Here's how the part is built. I have some questions about the finished solid (model axes, mm). Face numbers are marked on the shaded views. A direction names the side the tool comes from. Round coordinates to 2 decimals unless told otherwise and drop trailing zeros. Loops run counter-clockwise (first coordinate to the right, second up) from the corner with the lowest first, then second, coordinate; pieces in that order, holes last. Notation, with made-up numbers: (-11, 20) -> (19, 20) arc R26 ccw to (19, 57) -> close; hole circle Ø1 at (59.25, 8). An arc over 180 degrees is marked (long way). Use one line per item in the form item = value. Start each with the question number.
Item 1: If we section it at D-D (z = 210.5): Write out the boundary of the cut face in (x, y) (1 decimal).
Item 2: I'm going to push flat-ended pins straight in: pin 1 Ø1.5 at (x, y) = (-221, -40.5) entering from +Z (3 decimals); pin 2 Ø2.5 at (x, y) = (186.5, -3.5) entering from +Z (3 decimals); pin 3 Ø3 at (x, y) = (74.5, 52.5) entering from -Z. Where does each tip first touch, or does it pass through?
Item 3: Thinking about a two-plate mould opening in Y: for the marked faces 3, 4, 5 and 6, which applies, released by +Y, released by -Y, zero draft, split by the parting line, or undercut?
Item 4: If we section it at C-C (x = -102): Write out the boundary of the cut face in (y, z) (1 decimal).
Item 5: If we section it at A-A (z = 130.5): State how many separate pieces and enclosed holes the cut face has, then the cut area to 3 significant figures.
Item 6: If we section it at B-B (y = 84): Write out the boundary of the cut face in (x, z) (3 decimals), then the cut area to 3 significant figures.
Item 7: If I drill on L1, parallel to X at y = 47, z = 183 (3 decimals); L2, parallel to Y at x = -155, z = 75.5; L3, parallel to Z at x = 12, y = 120 (3 decimals), over which ranges is the centre line in solid material (lowest first)? Write a range as [from, to].
Item 8: For the marked faces 1 and 2, which set-ups out of +Z, -Z, +X, -X, +Y, -Y let a thin tool reach every point of the face, with its end or its side?
```python
from build123d import *

# Parameters (mm, degrees)
SKETCH1_W           = 558.8
SKETCH1_H           = 315.575
SKETCH1_W_2         = 552.45
SKETCH1_H_2         = 309.225
SKETCH1_W_3         = 3.175
SKETCH1_W_4         = 89.789
SKETCH1_W_5         = 88.775
SKETCH1_W_6         = 88.644
BOSS_EXTRUDE1_DEPTH = 3.175
SKETCH2_W           = 558.8
SKETCH2_H           = 315.575
SKETCH2_W_2         = 552.45
SKETCH2_H_2         = 309.225
SKETCH2_W_3         = 3.175
BOSS_EXTRUDE2_DEPTH = 200.6
SKETCH3_W           = 558.8
SKETCH3_H           = 315.575
BOSS_EXTRUDE3_DEPTH = 32
CUT_EXTRUDE1_DEPTH  = 483.951127186


with BuildPart() as part:
    # Sketch1 → Boss-Extrude1 (new body)
    # profile 1 of 12: a face of its own
    with BuildSketch(Plane.XY):
        Rectangle(SKETCH1_W, SKETCH1_H)
        Rectangle(SKETCH1_W_2, SKETCH1_H_2, mode=Mode.SUBTRACT)
    # profile 2 of 12: a face of its own
    with BuildSketch(Plane.XY):
        with Locations((-185.8625, 0)):
            Rectangle(SKETCH1_W_3, SKETCH1_H_2)
    # profile 3 of 12: a face of its own
    with BuildSketch(Plane.XY):
        with Locations((-139.3805, 0)):
            Rectangle(SKETCH1_W_4, SKETCH1_H_2)
    # profile 4 of 12: a face of its own
    with BuildSketch(Plane.XY):
        with Locations((-231.8375, 0)):
            Rectangle(SKETCH1_W_5, SKETCH1_H_2)
    # profile 5 of 12: a face of its own
    with BuildSketch(Plane.XY):
        with Locations((-46.4165, 0)):
            Rectangle(SKETCH1_W_4, SKETCH1_H_2)
    # profile 6 of 12: a face of its own
    with BuildSketch(Plane.XY):
        with Locations((-92.8985, 0)):
            Rectangle(SKETCH1_W_3, SKETCH1_H_2)
    # profile 7 of 12: a face of its own
    with BuildSketch(Plane.XY):
        with Locations((46.5475, 0)):
            Rectangle(SKETCH1_W_4, SKETCH1_H_2)
    # profile 8 of 12: a face of its own
    with BuildSketch(Plane.XY):
        with Locations((0.0655, 0)):
            Rectangle(SKETCH1_W_3, SKETCH1_H_2)
    # profile 9 of 12: a face of its own
    with BuildSketch(Plane.XY):
        with Locations((139.5115, 0)):
            Rectangle(SKETCH1_W_4, SKETCH1_H_2)
    # profile 10 of 12: a face of its own
    with BuildSketch(Plane.XY):
        with Locations((93.0295, 0)):
            Rectangle(SKETCH1_W_3, SKETCH1_H_2)
    # profile 11 of 12: a face of its own
    with BuildSketch(Plane.XY):
        with Locations((231.903, 0)):
            Rectangle(SKETCH1_W_6, SKETCH1_H_2)
    # profile 12 of 12: a face of its own
    with BuildSketch(Plane.XY):
        with Locations((185.9935, 0)):
            Rectangle(SKETCH1_W_3, SKETCH1_H_2)
    extrude(amount=BOSS_EXTRUDE1_DEPTH)

    # Sketch2 → Boss-Extrude2 (add)
    # profile 1 of 6: a face of its own
    with BuildSketch(Plane.XY.offset(3.175)):
        Rectangle(SKETCH2_W, SKETCH2_H)
        Rectangle(SKETCH2_W_2, SKETCH2_H_2, mode=Mode.SUBTRACT)
    # profile 2 of 6: a face of its own
    with BuildSketch(Plane.XY.offset(3.175)):
        with Locations((-185.8625, 0)):
            Rectangle(SKETCH2_W_3, SKETCH2_H_2)
    # profile 3 of 6: a face of its own
    with BuildSketch(Plane.XY.offset(3.175)):
        with Locations((-92.8985, 0)):
            Rectangle(SKETCH2_W_3, SKETCH2_H_2)
    # profile 4 of 6: a face of its own
    with BuildSketch(Plane.XY.offset(3.175)):
        with Locations((0.0655, 0)):
            Rectangle(SKETCH2_W_3, SKETCH2_H_2)
    # profile 5 of 6: a face of its own
    with BuildSketch(Plane.XY.offset(3.175)):
        with Locations((93.0295, 0)):
            Rectangle(SKETCH2_W_3, SKETCH2_H_2)
    # profile 6 of 6: a face of its own
    with BuildSketch(Plane.XY.offset(3.175)):
        with Locations((185.9935, 0)):
            Rectangle(SKETCH2_W_3, SKETCH2_H_2)
    extrude(amount=BOSS_EXTRUDE2_DEPTH)

    # Sketch3 → Boss-Extrude3 (add)
    with BuildSketch(Plane.XY.offset(203.775)):
        Rectangle(SKETCH3_W, SKETCH3_H)
        Polygon((187.581, 154.6125), (276.225, 154.6125), (276.225, -154.6125), (187.581, -154.6125), (184.406, -154.6125), (94.617, -154.6125), (91.442, -154.6125), (1.653, -154.6125), (-1.522, -154.6125), (-91.311, -154.6125), (-94.486, -154.6125), (-184.275, -154.6125), (-187.45, -154.6125), (-276.225, -154.6125), (-276.225, 154.6125), (-187.45, 154.6125), (-184.275, 154.6125), (-94.486, 154.6125), (-91.311, 154.6125), (-1.522, 154.6125), (1.653, 154.6125), (91.442, 154.6125), (94.617, 154.6125), (184.406, 154.6125), align=None, mode=Mode.SUBTRACT)
    extrude(amount=BOSS_EXTRUDE3_DEPTH)

    # Sketch4 → Cut-Extrude1 (cut, through all)
    with BuildSketch(Plane.XZ.offset(157.7875)):
        Polygon((279.4, 235.775), (209.4, 235.775), (279.4, 175.775), align=None)
    extrude(amount=-CUT_EXTRUDE1_DEPTH, mode=Mode.SUBTRACT)


solid = part.part
```
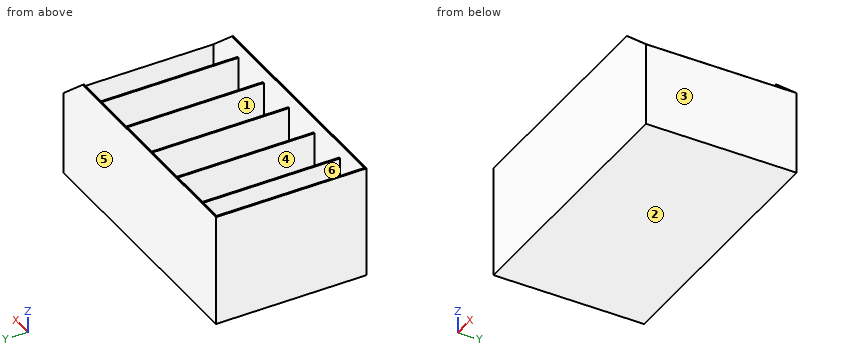
Values found:
q1.outline = (-279.4, -157.8) -> (238.9, -157.8) -> (238.9, -154.6) -> (-276.2, -154.6) -> (-276.2, 154.6) -> (238.9, 154.6) -> (238.9, 157.8) -> (-279.4, 157.8) -> close
q2.pin_1 = 3.175
q2.pin_2 = 203.775
q2.pin_3 = 0
q3.face_3 = zero draft
q3.face_4 = undercut
q3.face_5 = released by +Y
q3.face_6 = undercut
q4.outline = (-157.8, 0) -> (157.8, 0) -> (157.8, 235.8) -> (154.6, 235.8) -> (154.6, 3.2) -> (-154.6, 3.2) -> (-154.6, 235.8) -> (-157.8, 235.8) -> close
q5.separate_pieces = 1
q5.enclosed_holes = 6
q5.area = 10,400 mm2
q6.outline = (-279.4, 0) -> (279.4, 0) -> (279.4, 175.775) -> (276.225, 178.496) -> (276.225, 3.175) -> (187.581, 3.175) -> (187.581, 203.775) -> (184.406, 203.775) -> (184.406, 3.175) -> (94.617, 3.175) -> (94.617, 203.775) -> (91.442, 203.775) -> (91.442, 3.175) -> (1.653, 3.175) -> (1.653, 203.775) -> (-1.522, 203.775) -> (-1.522, 3.175) -> (-91.311, 3.175) -> (-91.311, 203.775) -> (-94.486, 203.775) -> (-94.486, 3.175) -> (-184.275, 3.175) -> (-184.275, 203.775) -> (-187.45, 203.775) -> (-187.45, 3.175) -> (-276.225, 3.175) -> (-276.225, 235.775) -> (-279.4, 235.775) -> close
q6.area = 6,250 mm2
q7.L1 = [-279.4, -276.225], [-187.45, -184.275], [-94.486, -91.311], [-1.522, 1.653], [91.442, 94.617], [184.406, 187.581]
q7.L2 = [-157.79, -154.61], [154.61, 157.79]
q7.L3 = [0, 3.175]
q8.face_1 = +Z
q8.face_2 = -Z, +X, -X, +Y, -Y
